The listing builds one solid part. Answer for the finished solid, in the listing's coordinates (mm). Face numbers are marked on the shaded views. Round coordinates to 2 decimals unless told otherwise and drop trailing zeros. Write each loop counter-clockwise with the first axis right and the second up, starting at its lowest first coordinate (ties: lowest second). Pieces come first, ordered by that corner, then holes. Notation, with made-up numbers: M 52,9.5 L 108,9.5 A13 cw 108,21.5 Z; hole C -39.75,66.25 d10. An arc over 180 degrees is marked long. One line per item, written item: value. Start each with the question number.
(1) Section B-B (y = 46.5) is taken. Determine the outline of the cut face in (x, z).
(2) Given P1, Ø0.9, axis at x = 60.5, y = 1.5, coming from the -Z side; P2, Ø10, axis at y = 20, z = -10.5, coming from the +X side; P3, Ø12, axis at x = 21.5, y = 15, coming from the +Z side, each flat-ended and moving along its own axis, determine where each tip first touches the part or whether it passes through.
(3) For a pull along X with two mould halves and no side action, classify the marked faces 1, 2 and 3 as released by +X, released by -X, zero draft, split by the parting line, or undercut.
(4) Consider probe 1 along X at (y, z) = (7, 6); probe 2 along X at (y, z) = (15.5, -11.5); probe 3 along Z at (x, y) = (-16.5, 27.5). Determine where each line is inside the solid, lowest interval first.
(5) Section D-D (y = 28.5) is taken. Determine the outline of the cut face in (x, z).
```python
from build123d import *

# Parameters (mm, degrees)
BOSS_EXTRUDE2_DEPTH = 3


with BuildPart() as part:
    # Sketch6 → Revolve1 (revolve)
    with BuildSketch(Plane(origin=(0, 0, 0), x_dir=(0, 0, -1), z_dir=(1, 0, 0)), mode=Mode.PRIVATE) as revolve1_sk:
        with BuildLine():
            Line((0, 0), (-20, 0))
            Line((-20, 0), (-25, 8.660254038))
            Line((-25, 8.660254038), (-25, 25))
            Line((-25, 25), (-23, 50))
            Line((-23, 50), (-22, 50))
            Line((-22, 50), (-24, 25))
            ThreePointArc((-24, 25), (-17.041420129, 7.900244501), (0, 0.8))
            Line((0, 0.8), (0, 0))
        make_face()
    revolve(revolve1_sk.sketch.rotate(Axis((0, 0.628504357, 0), (0, 1, 0)), 180), axis=Axis((0, 0.628504357, 0), (0, 1, 0)))

    # Sketch7 → Boss-Extrude2 (add)
    with BuildSketch(Plane(origin=(0, 0, 0), x_dir=(1, 0, 0), z_dir=(0, 1, 0))):
        with BuildLine():
            Line((23.887428117, -10), (80, -10))
            Line((80, -10), (80, 10))
            Line((80, 10), (23.887428117, 10))
            ThreePointArc((23.887428117, 10), (18.662529879, 11.049522995), (14.248195421, 14.035274392))
            ThreePointArc((14.248195421, 14.035274392), (20, 0), (14.248195421, -14.035274392))
            ThreePointArc((14.248195421, -14.035274392), (18.662529879, -11.049522995), (23.887428117, -10))
        make_face()
    extrude(amount=BOSS_EXTRUDE2_DEPTH)


solid = part.part
```
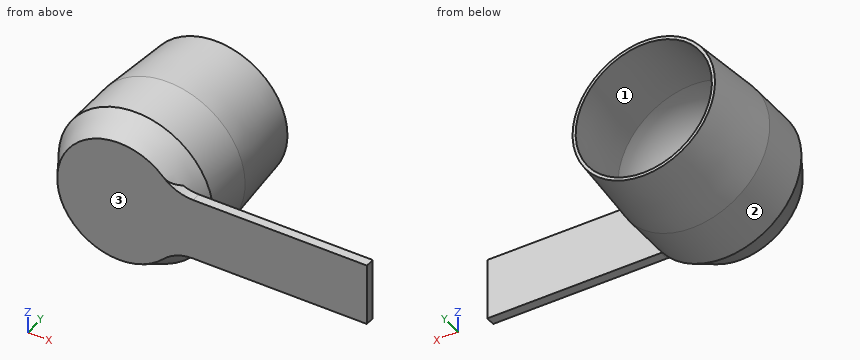
Recorded:
1. outline: C 0,0 d46.56; hole C 0,0 d44.56
2. P1: stops at z = -10
2. P2: stops at x = 24.39
2. P3: stops at z = 19.62
3. face 1: undercut
3. face 2: split by the parting line
3. face 3: zero draft
4. probe 1: x = -23.28 to -14.94, 14.94 to 23.28
4. probe 2: x = -22.2 to -18.9, 18.9 to 22.2
4. probe 3: z = -18.51 to -17.15, 17.15 to 18.51
5. outline: C 0,0 d49.44; hole C 0,0 d47.44
